from build123d import *

# Parameters (mm, degrees)
F0_R     = 4.445
F1_DEPTH = 8.89
F3_DEPTH = 6.35
F4_R     = 9.525
F5_DEPTH = 5.08
F6_R     = 5.07999


# Not quite as in the source:
# - a fillet or chamfer is up to 0.001 mm smaller than in the source, because OpenCascade refuses the exact size


with BuildPart() as f1:
    # F0 (on Top) → F1 (new body)
    with BuildSketch(Plane.XY):
        Circle(F0_R)
    extrude(amount=F1_DEPTH)

    # F2 (on face) → F3 (join)
    with BuildSketch(Plane.XY.offset(8.89)):
        with BuildLine():
            Line((-13.0288261443, -4.445), (11.0172175353, -4.445))
            ThreePointArc((11.0172175353, -4.445), (12.4023835963, -3.0598339389), (11.0172175353, -1.6746678779))
            Line((11.0172175353, -1.6746678779), (-4.1174643288, -1.6746678779))
            Line((-4.1174643288, -1.6746678779), (-13.0288261443, -1.6746678779))
            ThreePointArc((-13.0288261443, -1.6746678779), (-14.4139922054, -3.0598339389), (-13.0288261443, -4.445))
        make_face()
        with BuildLine():
            Line((-4.1174643288, -1.6746678779), (11.0172175353, -1.6746678779))
            ThreePointArc((11.0172175353, -1.6746678779), (8.99040904, 15.1069926007), (-6.8009194972, 9.0765677298))
            ThreePointArc((-6.8009194972, 9.0765677298), (-2.3607405432, 4.4743080446), (-4.1174643288, -1.6746678779))
        make_face()
        with BuildLine():
            ThreePointArc((-6.8009194972, 9.0765677298), (-14.1136776733, 6.1332066084), (-13.0288261443, -1.6746678779))
            Line((-13.0288261443, -1.6746678779), (-4.1174643288, -1.6746678779))
            ThreePointArc((-4.1174643288, -1.6746678779), (-6.9553513424, 3.3275159413), (-6.8009194972, 9.0765677298))
        make_face()
        with BuildLine():
            ThreePointArc((-6.8009194972, 9.0765677298), (-6.9553513424, 3.3275159413), (-4.1174643288, -1.6746678779))
            ThreePointArc((-4.1174643288, -1.6746678779), (-2.3607405432, 4.4743080446), (-6.8009194972, 9.0765677298))
        make_face()
    extrude(amount=F3_DEPTH)

    # F4 (on face) → F5 (join)
    with BuildSketch(Plane(origin=(0, 0, 0), x_dir=(1, 0, 0), z_dir=(0, 0, -1))):
        Circle(F4_R)
    extrude(amount=F5_DEPTH)

    # F6 (radius 5.08 in the source; OpenCascade refuses exactly that, so slightly less here)
    f6_edges = [f1.edges().sort_by_distance(p)[0] for p in [
        (-9.525, 0, -5.08),
    ]]
    fillet(f6_edges, radius=F6_R)


solid = f1.part
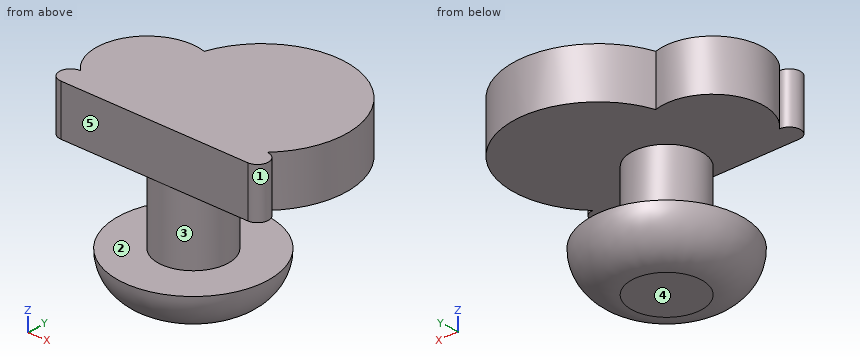
Geometry check sheet. Reference: the model listing, model coordinates, mm. Face numbers are marked on the shaded views. A direction names the side the tool comes from. Give positions to 0.01 mm unless a question says otherwise; leave off trailing zeros. Order: outer loops, then holes, each group sorted by start corner. A loop starts at its lowest first (then second) coordinate and runs counter-clockwise, first axis right, second up.
1. Sectioned sample at C-C (y = 11.5). Record the boundary of the cut face in (x, z), then the cut area to 3 significant figures.
Completed:
outline: (-5.71, 8.89) - (12.61, 8.89) - (12.61, 15.24) - (-5.71, 15.24) - close
area: 116 mm2
2. Sectioned sample at A-A (z = 8.5). Record the boundary of the cut face in (x, y) (3 decimals), then the cut area to 3 significant figures.
Completed:
outline: circle Ø8.89 at (0, 0)
area: 62.1 mm2
3. Depth check by flat-ended pin: pin 1 (6.5 mm diameter, centred on x = -7.5, y = 3, fed in from -Z); pin 2 (5 mm diameter, centred on y = -5, z = 3, fed in from -X); pin 3 (1 mm diameter, centred on x = 0, z = 2.5, fed in from +Y) (3 decimals). Enter the tip coordinate at first touch or a pass-through.
Completed:
pin 1: stops at z = -5.07
pin 2: stops at x = -3.68
pin 3: stops at y = 4.445
4. Draft check along Y on the marked faces 1, 2 and 3. Enter one of: pulls with the +Y half, pulls with the -Y half, needs draft (parallel to the pull), parting line crosses it, or undercut.
Completed:
face 1: undercut
face 2: needs draft
face 3: parting line crosses it
5. Access from +Z, -Z, +X, -X, +Y, -Y to the whole of each face (thin tool, end or side, straight path). Record for the marked faces 4 and 5.
Completed:
face 4: -Z, +X, -X, +Y, -Y
face 5: +Z, +X, -X, -Y
6. Sectioned sample at B-B (y = 14.5). Record the boundary of the cut face in (x, z).
Completed:
outline: (-2.99, 8.89) - (9.89, 8.89) - (9.89, 15.24) - (-2.99, 15.24) - close
7. Scan lines: line 1 (X direction, y = 0, z = 8.75) (3 decimals); line 2 (Z direction, x = 10.5, y = 0.5); line 3 (Y direction, x = -13.25, z = 10.75). Record each from-to range of solid material in increasing order.
Completed:
line 1: x = -4.445 to 4.445
line 2: z = 8.89 to 15.24
line 3: y = -4.43 to -1.69, -1.45 to 7.3
